Source: CAD feature listing. Evaluate the final solid. Frame: model axes, mm. Face numbers are marked on the shaded views. A direction names the side the tool comes from. Give positions to 0.01 mm unless a question says otherwise; leave off trailing zeros. Order: outer loops, then holes, each group sorted by start corner. A loop starts at its lowest first (then second) coordinate and runs counter-clockwise, first axis right, second up.
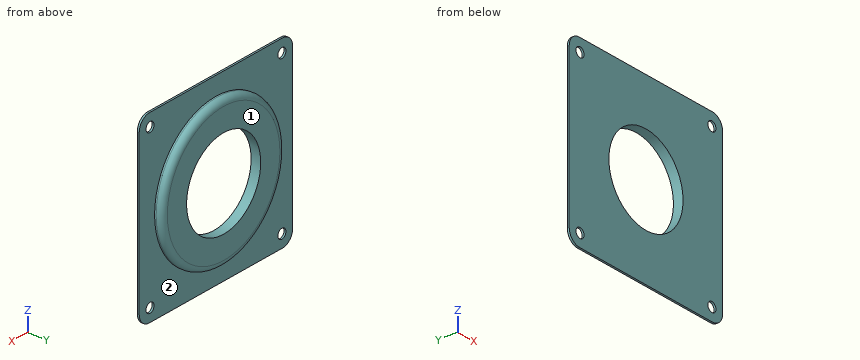
from build123d import *

# Parameters (mm, degrees)
SKETCH1_W           = 76.2
SKETCH1_H           = 76.2
SKETCH1_R           = 2.000000064
SKETCH1_R_2         = 18.415
BOSS_EXTRUDE1_DEPTH = 0.8
FILLET1_R           = 5.08
SKETCH2_R           = 30.48
SKETCH2_R_2         = 18.415
BOSS_EXTRUDE2_DEPTH = 3.2
FILLET2_R           = 2.54


with BuildPart() as part:
    # Sketch1 → Boss-Extrude1 (new body)
    with BuildSketch(Plane(origin=(0, 0, 0), x_dir=(1, 0, 0), z_dir=(0, 1, 0))):
        Rectangle(SKETCH1_W, SKETCH1_H)
        with Locations((-32.75, 32.75)):
            Circle(SKETCH1_R, mode=Mode.SUBTRACT)
        with Locations((32.75, 32.75)):
            Circle(SKETCH1_R, mode=Mode.SUBTRACT)
        with Locations((32.75, -32.75)):
            Circle(SKETCH1_R, mode=Mode.SUBTRACT)
        with Locations((-32.75, -32.75)):
            Circle(SKETCH1_R, mode=Mode.SUBTRACT)
        Circle(SKETCH1_R_2, mode=Mode.SUBTRACT)
    extrude(amount=BOSS_EXTRUDE1_DEPTH)

    # Fillet1
    fillet1_edges = [part.edges().sort_by_distance(p)[0] for p in [
        (38.1, 0.4, 38.1),
        (-38.1, 0.4, 38.1),
        (-38.1, 0.4, -38.1),
        (38.1, 0.4, -38.1),
    ]]
    fillet(fillet1_edges, radius=FILLET1_R)

    # Sketch2 → Boss-Extrude2 (add)
    with BuildSketch(Plane(origin=(0, 0.8, 0), x_dir=(1, 0, 0), z_dir=(0, 1, 0))):
        Circle(SKETCH2_R)
        Circle(SKETCH2_R_2, mode=Mode.SUBTRACT)
    extrude(amount=BOSS_EXTRUDE2_DEPTH)

    # Fillet2
    fillet2_edges = [part.edges().sort_by_distance(p)[0] for p in [
        (-30.48, 4, 0),
    ]]
    fillet(fillet2_edges, radius=FILLET2_R)


solid = part.part
1) Ray query, L1, parallel to Z at x = -32.75, y = 0.4; L2, parallel to X at y = 1.1, z = 0 (3 decimals). Return the intervals inside material, ascending.
Checks:
L1: z = -38.1 to -34.75, -30.75 to 30.75, 34.75 to 38.1
L2: x = -30.48 to -18.415, 18.415 to 30.48
2) Section query A-A on x = 0. Output: boundary loops of the cut face in (y, z) (3 decimals), and give its area (3 significant figures).
Checks:
outline: (0, -38.1) - (0.8, -38.1) - (0.8, -30.48) - (1.46, -30.48) arc R2.54 ccw to (4, -27.94) - (4, -18.415) - (0, -18.415) - close; (0, 18.415) - (4, 18.415) - (4, 27.94) arc R2.54 ccw to (1.46, 30.48) - (0.8, 30.48) - (0.8, 38.1) - (0, 38.1) - close
area: 106 mm2
3) First-contact query: pin 1 Ø1.5 at (x, y) = (-26, 2.5) entering from -Z; pin 2 Ø2 at (x, y) = (-1, 2.5) entering from -Z. Flat tips, straight axial feed; report the tip coordinate or a pass-through.
Checks:
pin 1: stops at z = -16.78
pin 2: stops at z = -30.47
4) Section query B-B on y = 2.5. Output: boundary loops of the cut face in (x, z) (3 decimals), and give its area (3 significant figures).
Checks:
outline: circle Ø60.515 at (0, 0); hole circle Ø36.83 at (0, 0)
area: 1,810 mm2
5) Reachability of the marked faces 1 and 2 from +Z, -Z, +X, -X, +Y, -Y: full face, straight path, thin tool, end or side. Return the list, or none.
Checks:
face 1: +Z, -Z, +X, -X, +Y
face 2: +Y
